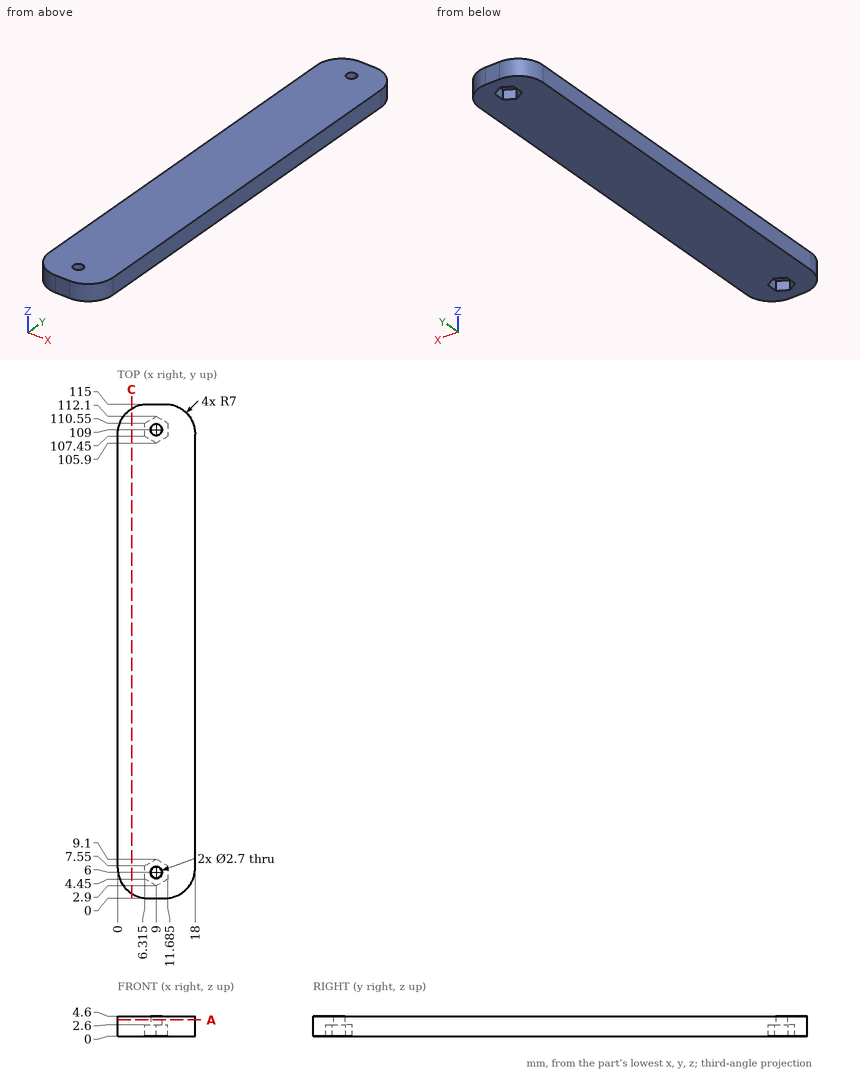
Answer from the drawing. Dimensions are ordinates in mm from the lowest x, y and z of the part. Round coordinates to 2 decimals unless told otherwise and drop trailing zeros. Write each loop counter-clockwise with the first axis right and the second up, starting at its lowest first coordinate (ties: lowest second). Pieces come first, ordered by that corner, then holes.
1. Straight lines are drawn through the part: L1, parallel to Y at x = 9, z = 3.15; L2, parallel to Y at x = 8, z = 3.7 (1 decimal); L3, parallel to X at y = 108.5, z = 1 (1 decimal). For each, find the intervals that lie inside material, in ascending order.
2. The part is cut by section A-A, the plane z = 3.75. Determine the outline of the cut face in (x, y), then the cut area to 3 significant figures.
3. Given pin 1 Ø2.5 at (x, y) = (9, 7.5) entering from -Z; pin 2 Ø0.8 at (y, z) = (109, 1) entering from +X; pin 3 Ø1 at (x, z) = (15, 3) entering from -Y; pin 4 Ø2.5 at (x, y) = (9, 6) entering from -Z, each flat-ended and moving along its own axis, determine where each tip first touches the part or whether it passes through.
4. The part is cut by section C-C, the plane x = 3.25. Determine the outline of the cut face in (y, z), then the cut area to 3 significant figures.
Values:
1. L1: y = 0 to 4.65, 7.35 to 107.65, 110.35 to 115
1. L2: y = 0 to 5.1, 6.9 to 108.1, 109.9 to 115
1. L3: x = 0 to 6.3, 11.7 to 18
2. outline: (0, 7) arc R7 ccw to (7, 0) - (11, 0) arc R7 ccw to (18, 7) - (18, 108) arc R7 ccw to (11, 115) - (7, 115) arc R7 ccw to (0, 108) - close; hole circle Ø2.7 at (9, 6); hole circle Ø2.7 at (9, 109)
2. area: 2,020 mm2
3. pin 1: stops at z = 2.6
3. pin 2: stops at x = 17.97
3. pin 3: stops at y = 0.94
3. pin 4: passes through
4. outline: (1.09, 0) - (113.91, 0) - (113.91, 4.6) - (1.09, 4.6) - close
4. area: 519 mm2
